Autodesk Inventor part; units mm, degrees
ref_plane "YZ Plane" through (0, 0, 0) normal (1, 0, 0) x (0, 1, 0)
ref_plane "XZ Plane" through (0, 0, 0) normal (0, 1, 0) x (-1, 0, 0)
ref_plane "XY Plane" through (0, 0, 0) normal (0, 0, 1) x (1, 0, 0)
sketch "Sketch1" plane through (0, 0, 0) normal (1, 0, 0) x (0, 1, 0)
  circle A0 centre (169.2255, 363.3555) radius 48.0965
  circle A1 centre (138.8493, 276.6293) radius 6.35
  point P0 (0, 0)
  dimension "d0" = 12.7
extrude "Extrusion1" add sketch "Sketch1" along normal blind 4.7625 contours A1
chamfer "Chamfer1" distance 3.175 angle 45 1 edges at (4.7625, 132.4993, 276.6293)
sketch "Sketch2" plane through (4.7625, 138.8493, 276.6293) normal (1, 0, 0) x (0, 0, -1)
  circle A0 centre (0, 0) radius 3.175
  circle A1 centre (0, 0) radius 3.175
  point P0 (276.6293, -138.8493)
extrude "Extrusion2" add sketch "Sketch2" along normal blind 22.225
chamfer "Chamfer2" distance 3.175 angle 45 1 edges at (26.9875, 138.8493, 279.8043)
sketch "Sketch3" plane through (0, 138.8493, 276.6293) normal (-1, 0, 0) x (0, 0, 1)
  point P0 (-276.6293, -138.8493)
thread "Thread1"
sketch "Sketch4" plane through (0, 138.8493, 276.6293) normal (-1, 0, 0) x (0, 0, 1)
  line L0 (-1.16, 5.6468) -> (1.058, 5.6468)
  line L1 (1.058, 5.6468) -> (1.058, -5.4225)
  line L2 (1.058, -5.4225) -> (-1.16, -5.4225)
  line L3 (-1.16, -5.4225) -> (-1.16, 5.6468)
  line L4 (-5.2022, 1.2937) -> (5.5977, 1.2937)
  line L5 (5.5977, 1.2937) -> (5.5977, -1.1109)
  line L6 (5.5977, -1.1109) -> (-5.2022, -1.1109)
  line L7 (-5.2022, -1.1109) -> (-5.2022, 1.2937)
  point P0 (-276.6293, -138.8493)
extrude "Extrusion3" cut sketch "Sketch4" against normal blind 3.175
properties part number "screw"
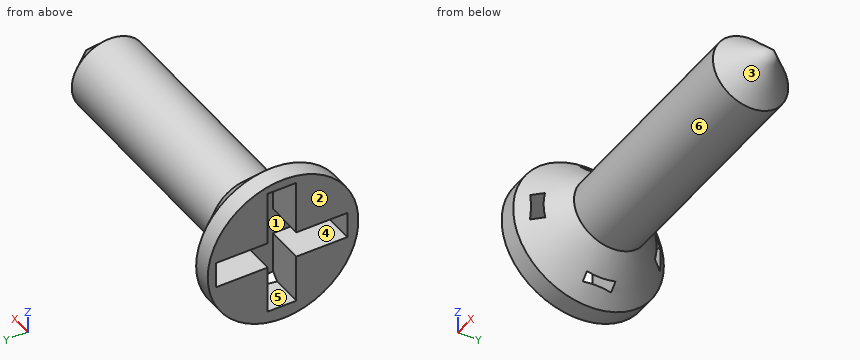
CAD build for the part. Positions are in the model's coordinates, mm. Face numbers are marked on the shaded views. A direction names the side the tool comes from. Round coordinates to 2 decimals unless told otherwise and drop trailing zeros. Order: outer loops, then holes, each group sorted by start corner. A loop starts at its lowest first (then second) coordinate and runs counter-clockwise, first axis right, second up. Notation, with made-up numbers: (61, -33.5) -> (97, -33.5) arc R14 ccw to (97, -21.5) -> close; hole circle Ø3 at (62.5, 64). An arc over 180 degrees is marked (long way). One line per question, with ' | ' between items.
Q1. Two-plate mould, pull along Z, no slides. Class the marked faces 1, 2 and 3: released by +Z, released by -Z, zero draft, split by the parting line, or undercut.
Completed:
face 1: undercut | face 2: zero draft | face 3: split by the parting line
Q2. Slice it at A-A (y = 139.5). Give the number of separate pieces and of enclosed holes in the cut face, then the cut area to 3 significant figures.
Completed:
separate pieces: 3 | enclosed holes: 0 | area: 144 mm^2
Q3. Which spindle directions (+Z, -Z, +X, -X, +Y, -Y) get a long thin tool onto all of the face, cutting with end or side? Do the marked faces 4, 5 and 6. Say none if no direction does.
Completed:
face 4: -X | face 5: +X, -X | face 6: +X
Q4. Probe probe 1 along Y at (x, z) = (21.5, 276.5); probe 2 along Y at (x, z) = (1.5, 278.25); probe 3 along X at (y, z) = (139.25, 271). List the from-to ranges inside material, lowest first.
Completed:
probe 1: y = 135.68 to 142.02 | probe 2: y = 132.71 to 137.74, 140.14 to 144.99 | probe 3: x = 0 to 2.29
Q5. Slice it at C-C (x = 12.25). Write the cut outline in (y, z) (3 decimals), then the cut area to 3 significant figures.
Completed:
outline: circle Ø6.35 at (138.849, 276.629) | area: 31.7 mm^2
Q6. Slice it at B-B (x = 3.5). Write the cut outline in (y, z) (1 decimal).
Completed:
outline: circle Ø8.9 at (138.8, 276.6)
Q7. Drop flat-ended pins along their axis: pin 1 (5 mm diameter, centred on x = 15.5, z = 278.5, fed in from -Y); pin 2 (1.5 mm diameter, centred on x = 11.5, y = 136, fed in from +Z); pin 3 (4 mm diameter, centred on x = 6, z = 274, fed in from +Y). Give the stop position or say it passes through.
Completed:
pin 1: stops at y = 135.67 | pin 2: stops at z = 279.01 | pin 3: stops at y = 142.15
